from build123d import *

# Parameters (mm, degrees)
SKETCH2_W           = 8
SKETCH2_H           = 30
BOSS_EXTRUDE1_DEPTH = 28
CUT_EXTRUDE1_REACH  = 52
SKETCH3_R           = 2.9
FILLET1_R           = 5
FILLET2_R           = 3
FILLET3_R           = 1
FILLET4_R           = 1
SKETCH4_W           = 7
SKETCH4_H           = 7
CUT_EXTRUDE2_DEPTH  = 20


with BuildPart() as part:
    # Sketch1 → Revolve1 (revolve)
    with BuildSketch(Plane.XY):
        Polygon((0, 0), (0, 24), (-29, 24), (-50, 3), (-50, 0), align=None)
    revolve(axis=Axis((0, 0, 0), (0, 1, 0)))

    # Sketch2 → Boss-Extrude1 (add)
    with BuildSketch(Plane(origin=(0, 24, 0), x_dir=(1, 0, 0), z_dir=(0, 1, 0))):
        with Locations((-12, 0)):
            Rectangle(SKETCH2_W, SKETCH2_H)
    extrude(amount=BOSS_EXTRUDE1_DEPTH)

    # Sketch3 → Cut-Extrude1 (cut, up to next)
    with BuildSketch(Plane(origin=(0, 0, 0), x_dir=(0, 0, -1), z_dir=(1, 0, 0)), mode=Mode.PRIVATE) as cut_extrude1_sk1:
        with Locations((-6.5, 46)):
            Circle(SKETCH3_R)
    cut_extrude1_tool1 = extrude(cut_extrude1_sk1.sketch, amount=-CUT_EXTRUDE1_REACH, mode=Mode.PRIVATE) & part.part
    add(cut_extrude1_tool1.solids().sort_by_distance((0, 46, 6.5))[0], mode=Mode.SUBTRACT)
    # Sketch3 → Cut-Extrude1 (cut, up to next)
    with BuildSketch(Plane(origin=(0, 0, 0), x_dir=(0, 0, -1), z_dir=(1, 0, 0)), mode=Mode.PRIVATE) as cut_extrude1_sk2:
        with Locations((6.5, 46)):
            Circle(SKETCH3_R)
    cut_extrude1_tool2 = extrude(cut_extrude1_sk2.sketch, amount=-CUT_EXTRUDE1_REACH, mode=Mode.PRIVATE) & part.part
    add(cut_extrude1_tool2.solids().sort_by_distance((0, 46, -6.5))[0], mode=Mode.SUBTRACT)

    # Fillet1
    fillet1_edges = [part.edges().sort_by_distance(p)[0] for p in [
        (-12, 52, 15),
        (-12, 52, -15),
    ]]
    fillet(fillet1_edges, radius=FILLET1_R)

    # Fillet2
    fillet2_edges = [part.edges().sort_by_distance(p)[0] for p in [
        (29, 24, 0),
    ]]
    fillet(fillet2_edges, radius=FILLET2_R)

    # Fillet3
    fillet3_edges = [part.edges().sort_by_distance(p)[0] for p in [
        (50, 3, 0),
    ]]
    fillet(fillet3_edges, radius=FILLET3_R)

    # Fillet4
    fillet4_edges = [part.edges().sort_by_distance(p)[0] for p in [
        (-16, 24, 0),
        (-12, 24, 15),
        (-8, 24, 0),
        (-12, 24, -15),
        (-16, 52, 0),
        (-8, 52, 0),
        (-16, 35.5, 15),
        (-16, 35.5, -15),
        (-16, 50.535533906, 13.535533906),
        (-16, 50.535533906, -13.535533906),
        (-8, 35.5, -15),
        (-8, 35.5, 15),
        (-8, 50.535533906, 13.535533906),
        (-8, 50.535533906, -13.535533906),
    ]]
    fillet(fillet4_edges, radius=FILLET4_R)

    # Sketch4 → Cut-Extrude2 (cut)
    with BuildSketch(Plane(origin=(0, 24, 0), x_dir=(1, 0, 0), z_dir=(0, 1, 0))):
        Rectangle(SKETCH4_W, SKETCH4_H)
    extrude(amount=-CUT_EXTRUDE2_DEPTH, mode=Mode.SUBTRACT)


solid = part.part
Read the model definition and answer for the solid it produces. Units are mm, in the model's axes. A direction names the side the tool comes from. Give positions to 0.01 mm unless a question says otherwise; leave off trailing zeros. Loops run counter-clockwise (first coordinate to the right, second up) from the corner with the lowest first, then second, coordinate; pieces in that order, holes last. Notation, with made-up numbers: (42, 24.5) - (96, 24.5) arc R9 cw to (96, 29.5) - close; hole circle Ø2 at (39.5, 0.5). An arc over 180 degrees is marked (long way). Answer as CSV lines item,"result". Start each with the question number.
1) Find section A-A (y = 44.5). Write down the section's boundary in (x, z).
2) Find section B-B (y = 30.5). Write down the section's boundary in (x, z).
3) Each of these flat-tipped pins is pushed along its axis until it touches: pin 1 Ø2 at (x, z) = (34, 28) entering from +Y; pin 2 Ø10 at (y, z) = (23, 10) entering from -X; pin 3 Ø7.5 at (x, y) = (0, 10.5) entering from +Z; pin 4 Ø12 at (y, z) = (31, 21.5) entering from +X. Where does it stop, or does it pass through?
4) Determine the mould class of faces 1 (the face through (-12, 36, 15)), 2 (the face through (-11.94, 43.17, 7.13)), 3 (the face through (-12, 52, 0)) for opening direction Z: released by +Z, released by -Z, zero draft, split by the parting line, or undercut.
5) Straight lines are drawn through the part: L1, parallel to Y at x = -10.25, z = 6.5; L2, parallel to Y at x = -4.5, z = 5.5; L3, parallel to X at y = 36, z = -4. For each, find the intervals that lie inside material, in ascending order. Write a range as from..to.
6) Which of the six approach directions +Z, -Z, +X, -X, +Y, -Y give full straight-line access (tool end or side, diameter ignored) to faces 4 (the face through (-8, 38, 0)), 5 (the face through (0, 14, -3.5)), 6 (the face through (-12, 36, -15))?
Findings below:
1,outline,"(-16, -14) arc R1 ccw to (-15, -15) - (-9, -15) arc R1 ccw to (-8, -14) - (-8, -8.98) - (-16, -8.98) - close; (-16, -4.02) - (-8, -4.02) - (-8, 4.02) - (-16, 4.02) - close; (-16, 8.98) - (-8, 8.98) - (-8, 14) arc R1 ccw to (-9, 15) - (-15, 15) arc R1 ccw to (-16, 14) - close"
2,outline,"(-16, -14) arc R1 ccw to (-15, -15) - (-9, -15) arc R1 ccw to (-8, -14) - (-8, 14) arc R1 ccw to (-9, 15) - (-15, 15) arc R1 ccw to (-16, 14) - close"
3,pin 1,"y = 9.95"
3,pin 2,"x = -33.72"
3,pin 3,"z = 46.25"
3,pin 4,"through"
4,face 1,"released by +Z"
4,face 2,"undercut"
4,face 3,"zero draft"
5,L1,"0..43.1, 48.9..52"
5,L2,"0..24"
5,L3,"-16..-8"
6,face 4,"+Z, -Z, +X, +Y"
6,face 5,"+Y"
6,face 6,"-Z, +X, -X, +Y"
